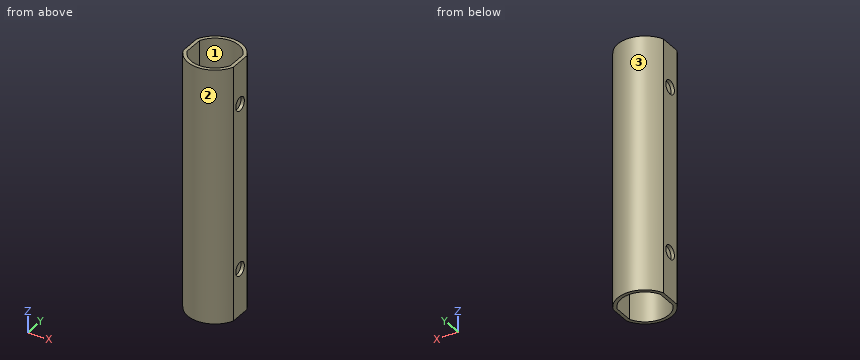
```python
from build123d import *

# Parameters (mm, degrees)
BOSS_EXTRUDE1_DEPTH = 117.85
CUT_EXTRUDE1_REACH  = 122.81
SKETCH2_R           = 3.175


with BuildPart() as part:
    # Sketch1 → Boss-Extrude1 (new body)
    with BuildSketch(Plane.XY):
        with BuildLine():
            Line((11.674330816, 5), (11.674330816, -5))
            ThreePointArc((11.674330816, -5), (0, -12.7), (-11.674330816, -5))
            Line((-11.674330816, -5), (-11.674330816, 5))
            ThreePointArc((-11.674330816, 5), (0, 12.7), (11.674330816, 5))
        make_face()
        with BuildLine():
            Line((10.086830816, 4.662992638), (10.086830816, -4.662992638))
            ThreePointArc((10.086830816, -4.662992638), (0, -11.1125), (-10.086830816, -4.662992638))
            Line((-10.086830816, -4.662992638), (-10.086830816, 4.662992638))
            ThreePointArc((-10.086830816, 4.662992638), (0, 11.1125), (10.086830816, 4.662992638))
        make_face(mode=Mode.SUBTRACT)
    extrude(amount=BOSS_EXTRUDE1_DEPTH)

    # Cut-Extrude1: up to this face of the body (flat: up to its plane)
    cut_extrude1_end = Plane(part.part.faces().sort_by_distance((-11.674330816, 0, 58.925))[0])
    # Sketch2 → Cut-Extrude1 (cut, up to the picked face)
    with BuildSketch(Plane(origin=(11.674330816, 0, 0), x_dir=(0, 0, -1), z_dir=(1, 0, 0)), mode=Mode.PRIVATE) as cut_extrude1_sk1:
        with Locations((-21.5, 0)):
            Circle(SKETCH2_R)
    cut_extrude1_tool1 = split(extrude(cut_extrude1_sk1.sketch, amount=-CUT_EXTRUDE1_REACH, mode=Mode.PRIVATE), bisect_by=cut_extrude1_end, keep=Keep.BOTH, mode=Mode.PRIVATE)
    # Sketch2 → Cut-Extrude1 (cut, up to the picked face)
    with BuildSketch(Plane(origin=(11.674330816, 0, 0), x_dir=(0, 0, -1), z_dir=(1, 0, 0)), mode=Mode.PRIVATE) as cut_extrude1_sk2:
        with Locations((-98.1, 0)):
            Circle(SKETCH2_R)
    cut_extrude1_tool2 = split(extrude(cut_extrude1_sk2.sketch, amount=-CUT_EXTRUDE1_REACH, mode=Mode.PRIVATE), bisect_by=cut_extrude1_end, keep=Keep.BOTH, mode=Mode.PRIVATE)
    add(cut_extrude1_tool1.solids().sort_by(Axis((11.674331, 0, 21.5), (-1, 0, 0)))[0], mode=Mode.SUBTRACT)
    add(cut_extrude1_tool2.solids().sort_by(Axis((11.674331, 0, 98.1), (-1, 0, 0)))[0], mode=Mode.SUBTRACT)


solid = part.part
```
Geometry check sheet. Reference: the model listing, model coordinates, mm. Face numbers are marked on the shaded views. Coordinates: 2 decimals unless noted, no trailing zeros. Loops run counter-clockwise (first coordinate to the right, second up) from the corner with the lowest first, then second, coordinate; pieces in that order, holes last.
Item 1: Thickness scan on line 1 (X direction, y = 0.5, z = 112); line 2 (Y direction, x = -7.5, z = 49.5); line 3 (Y direction, x = 2, z = 10). Record the ranges inside material, lowest first.
Item 2: Sectioned sample at D-D, the plane y = -2. Record the boundary of the cut face in (x, z).
Item 3: Sectioned sample at A-A, the plane z = 21.5. Record the boundary of the cut face in (x, y) (1 decimal).
Item 4: Sectioned sample at C-C, the plane z = 36.5. Record the boundary of the cut face in (x, y) (1 decimal).
Item 5: Release check for a two-part mould opening along Y. For the marked faces 1, 2 and 3 record: released by +Y, released by -Y, zero draft, split by the parting line, or undercut.
Item 6: Go/stop test with flat-tipped pins: pin 1 Ø3 at (x, z) = (-3, 50) entering from -Y; pin 2 Ø8.5 at (y, z) = (0, 21.5) entering from -X; pin 3 Ø1.5 at (y, z) = (-7.5, 70.5) entering from -X; pin 4 Ø5 at (x, z) = (-3.5, 32.5) entering from -Y. Record where each tip stops, or that it passes through.
Item 7: Sectioned sample at B-B, the plane x = 2. Record the boundary of the cut face in (y, z), then the cut area to 3 significant figures.
Check result:
1. line 1: x = -11.67 to -10.09, 10.09 to 11.67
1. line 2: y = -10.25 to -8.2, 8.2 to 10.25
1. line 3: y = -12.54 to -10.93, 10.93 to 12.54
2. outline: (-11.67, 0) - (-10.09, 0) - (-10.09, 19.03) - (-11.67, 19.03) - close; (-11.67, 23.97) - (-10.09, 23.97) - (-10.09, 95.63) - (-11.67, 95.63) - close; (-11.67, 100.57) - (-10.09, 100.57) - (-10.09, 117.85) - (-11.67, 117.85) - close; (10.09, 0) - (11.67, 0) - (11.67, 19.03) - (10.09, 19.03) - close; (10.09, 23.97) - (11.67, 23.97) - (11.67, 95.63) - (10.09, 95.63) - close; (10.09, 100.57) - (11.67, 100.57) - (11.67, 117.85) - (10.09, 117.85) - close
3. outline: (-11.7, -5) arc R12.7 ccw to (11.7, -5) - (11.7, -3.2) - (10.1, -3.2) - (10.1, -4.7) arc R11.1 cw to (-10.1, -4.7) - (-10.1, -3.2) - (-11.7, -3.2) - close; (-11.7, 3.2) - (-10.1, 3.2) - (-10.1, 4.7) arc R11.1 cw to (10.1, 4.7) - (10.1, 3.2) - (11.7, 3.2) - (11.7, 5) arc R12.7 ccw to (-11.7, 5) - close
4. outline: (-11.7, -5) arc R12.7 ccw to (11.7, -5) - (11.7, 5) arc R12.7 ccw to (-11.7, 5) - close; hole (-10.1, -4.7) arc R11.1 ccw to (10.1, -4.7) - (10.1, 4.7) arc R11.1 ccw to (-10.1, 4.7) - close
5. face 1: undercut
5. face 2: released by -Y
5. face 3: released by +Y
6. pin 1: stops at y = -12.61
6. pin 2: stops at x = -11.67
6. pin 3: stops at x = -10.76
6. pin 4: stops at y = -12.66
7. outline: (-12.54, 0) - (-10.93, 0) - (-10.93, 117.85) - (-12.54, 117.85) - close; (10.93, 0) - (12.54, 0) - (12.54, 117.85) - (10.93, 117.85) - close
7. area: 380 mm2
